The listing builds one solid part. Answer for the finished solid, in the listing's coordinates (mm). Round coordinates to 2 decimals unless told otherwise and drop trailing zeros. Order: outer loops, then holes, each group sorted by start corner. A loop starts at its lowest first (then second) coordinate and runs counter-clockwise, first axis right, second up. Notation, with made-up numbers: (-24, 72) - (17, 72) arc R16 ccw to (17, 77) - close; hole circle Ø11 at (81, -16). An arc over 180 degrees is marked (long way). Write item = value, one per line.
from build123d import *

# Parameters (mm, degrees)
ESQUISSE1_W                    = 390
ESQUISSE1_H                    = 65
BOSS_EXTRU_1_DEPTH             = 5
ESQUISSE2_W                    = 30
ESQUISSE2_H                    = 5
ENL_V_MAT_EXTRU_1_DEPTH        = 5
R_P_TITION_LIN_AIRE1_COUNT     = 6
R_P_TITION_LIN_AIRE1_PITCH     = 60
ESQUISSE3_W                    = 5
ESQUISSE3_H                    = 13
ENL_V_MAT_EXTRU_2_DEPTH        = 5
R_P_TITION_LIN_AIRE2_COUNT     = 2
R_P_TITION_LIN_AIRE2_PITCH     = 26
SYM_TRIE1_COPY_1_SKETCH_W      = 5
SYM_TRIE1_COPY_1_SKETCH_H      = 13
SYM_TRIE1_COPY_1_DEPTH         = 5
ESQUISSE4_R                    = 4
ENL_V_MAT_EXTRU_3_DEPTH        = 5
R_P_TITION_LIN_AIRE3_COUNT     = 10
R_P_TITION_LIN_AIRE3_PITCH     = 27.5
R_P_TITION_LIN_AIRE3_COL_COUNT = 3
R_P_TITION_LIN_AIRE3_COL_PITCH = 27.5
ESQUISSE5_W                    = 5
ESQUISSE5_H                    = 13
ESQUISSE5_W_2                  = 13
ESQUISSE5_H_2                  = 5
ENL_V_MAT_EXTRU_4_DEPTH        = 5
R_P_TITION_LIN_AIRE4_COUNT     = 3
R_P_TITION_LIN_AIRE4_PITCH     = 27.5
R_P_TITION_LIN_AIRE4_COL_COUNT = 11
R_P_TITION_LIN_AIRE4_COL_PITCH = 27.5


with BuildPart() as part:
    # Esquisse1 → Boss.-Extru.1 (new body)
    with BuildSketch(Plane.XY):
        with Locations((195, -32.5)):
            Rectangle(ESQUISSE1_W, ESQUISSE1_H)
    extrude(amount=BOSS_EXTRU_1_DEPTH)

    # Esquisse2 → Enlèv. mat.-Extru.1 (cut)
    with BuildSketch(Plane.XY.offset(5)):
        with Locations((45, -62.5)):
            Rectangle(ESQUISSE2_W, ESQUISSE2_H)
    enl_v_mat_extru_1 = extrude(amount=-ENL_V_MAT_EXTRU_1_DEPTH, mode=Mode.SUBTRACT)

    # Répétition linéaire1: Enlèv. mat.-Extru.1 ×6
    with Locations(*[(i * R_P_TITION_LIN_AIRE1_PITCH, 0, 0) for i in range(1, R_P_TITION_LIN_AIRE1_COUNT)]):
        add(enl_v_mat_extru_1, mode=Mode.SUBTRACT)

    # Esquisse3 → Enlèv. mat.-Extru.2 (cut)
    with BuildSketch(Plane.XY.offset(5)):
        with Locations((2.5, -45.5)):
            Rectangle(ESQUISSE3_W, ESQUISSE3_H)
    enl_v_mat_extru_2 = extrude(amount=-ENL_V_MAT_EXTRU_2_DEPTH, mode=Mode.SUBTRACT)

    # Répétition linéaire2: Enlèv. mat.-Extru.2 ×2
    with Locations(*[(0, i * R_P_TITION_LIN_AIRE2_PITCH, 0) for i in range(1, R_P_TITION_LIN_AIRE2_COUNT)]):
        add(enl_v_mat_extru_2, mode=Mode.SUBTRACT)

    # Symétrie1: Enlèv. mat.-Extru.2 across plane
    add(enl_v_mat_extru_2.mirror(Plane.ZY.offset(-195)), mode=Mode.SUBTRACT)

    # Symétrie1 copy 1 sketch → Symétrie1 copy 1 (cut)
    with BuildSketch(Plane(origin=(390, 26, 5), x_dir=(-1, 0, 0), z_dir=(0, 0, 1))):
        with Locations((2.5, 45.5)):
            Rectangle(SYM_TRIE1_COPY_1_SKETCH_W, SYM_TRIE1_COPY_1_SKETCH_H)
    extrude(amount=-SYM_TRIE1_COPY_1_DEPTH, mode=Mode.SUBTRACT)

    # Esquisse4 → Enlèv. mat.-Extru.3 (cut)
    with BuildSketch(Plane.XY.offset(5)):
        with Locations((100, -53)):
            Circle(ESQUISSE4_R)
    enl_v_mat_extru_3 = extrude(amount=-ENL_V_MAT_EXTRU_3_DEPTH, mode=Mode.SUBTRACT)

    # Répétition linéaire3: Enlèv. mat.-Extru.3 ×10
    with Locations(*[(i * R_P_TITION_LIN_AIRE3_PITCH, 0, 0) for i in range(1, R_P_TITION_LIN_AIRE3_COUNT)]):
        add(enl_v_mat_extru_3, mode=Mode.SUBTRACT)

    # Répétition linéaire3 col: Enlèv. mat.-Extru.3 ×3
    with Locations(*[(-i * R_P_TITION_LIN_AIRE3_COL_PITCH, 0, 0) for i in range(1, R_P_TITION_LIN_AIRE3_COL_COUNT)]):
        add(enl_v_mat_extru_3, mode=Mode.SUBTRACT)

    # Esquisse5 → Enlèv. mat.-Extru.4 (cut)
    with BuildSketch(Plane.XY.offset(5)):
        with Locations((86.25, -36.5)):
            Rectangle(ESQUISSE5_W, ESQUISSE5_H)
        with Locations((86.25, -18)):
            Rectangle(ESQUISSE5_W_2, ESQUISSE5_H_2)
    enl_v_mat_extru_4 = extrude(amount=-ENL_V_MAT_EXTRU_4_DEPTH, mode=Mode.SUBTRACT)

    # Répétition linéaire4: Enlèv. mat.-Extru.4 ×3
    with Locations(*[(-i * R_P_TITION_LIN_AIRE4_PITCH, 0, 0) for i in range(1, R_P_TITION_LIN_AIRE4_COUNT)]):
        add(enl_v_mat_extru_4, mode=Mode.SUBTRACT)

    # Répétition linéaire4 col: Enlèv. mat.-Extru.4 ×11
    with Locations(*[(i * R_P_TITION_LIN_AIRE4_COL_PITCH, 0, 0) for i in range(1, R_P_TITION_LIN_AIRE4_COL_COUNT)]):
        add(enl_v_mat_extru_4, mode=Mode.SUBTRACT)


solid = part.part
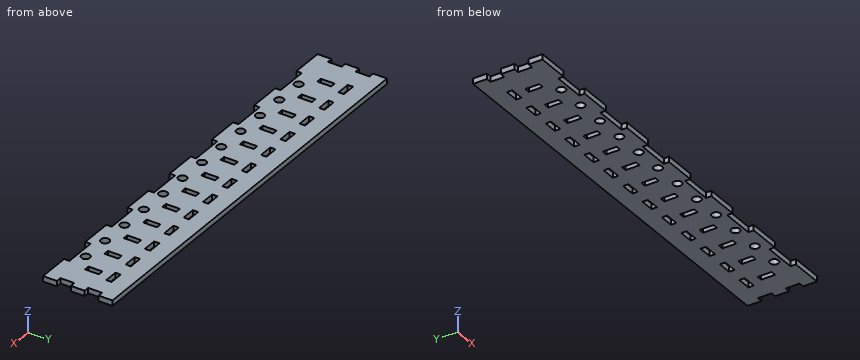
Q1. Flat-ended cylindrical pins translate along their axes: P1, Ø1.5, axis at y = -19, z = 3, coming from the +X side; P2, Ø1, axis at y = -44, z = 1, coming from the -X side; P3, Ø1.5, axis at x = 360.5, z = 2.5, coming from the +Y side; P4, Ø2.5, axis at x = 168.5, z = 3, coming from the -Y side. Find the tip coordinate at first contact, or state that the pin passes through.
Model answer:
P1 = 385
P2 = 5
P3 = 0
P4 = -60
Q2. Find the intervals of material crossed by line 1 (Y direction, x = 166.5, z = 4.85); line 2 (Y direction, x = 72.5, z = 3.7); line 3 (Y direction, x = 86, z = 2.2), in increasing order. Write a range as from..to.
Model answer:
line_1 = -60..-43, -30..-20.5, -15.5..0
line_2 = -65..-57, -49..0
line_3 = -65..-43, -30..-20.5, -15.5..0
Q3. Section A-A on x = 127.5 is taken. Determine the outline of the cut face in (y, z).
Model answer:
outline = (-65, 0) - (-57, 0) - (-57, 5) - (-65, 5) - close; (-49, 0) - (0, 0) - (0, 5) - (-49, 5) - close
Q4. Section B-B on z = 3.85 is taken. Count the separate pieces of the cut face and the enclosed holes in it, then the cut area to 3 significant figures.
Model answer:
separate_pieces = 1
enclosed_holes = 38
area = 21,900 mm^2
